from build123d import *

# Parameters (mm, degrees)
F0_W     = 40
F0_H     = 40
F1_DEPTH = 40.3
F2_W     = 25
F2_H     = 15
F3_DEPTH = 24.6
F6_W     = 20.776337
F6_H     = 21.012508
F7_DEPTH = 32
F8_R     = 7.245927
F8_R_2   = 6.636752
F8_R_3   = 8.331711
F8_R_4   = 4.708623
F9_DEPTH = 21.6


with BuildPart() as f1:
    # F0 (on Top) → F1 (new body)
    with BuildSketch(Plane.XY):
        with Locations((-31.879965, 27.884198)):
            Rectangle(F0_W, F0_H)
    extrude(amount=F1_DEPTH)

    # F2 (on face) → F3 (join)
    with BuildSketch(Plane.XZ.offset(-7.884198)):
        with Locations((-37.312957, 7.5)):
            Rectangle(F2_W, F2_H)
    extrude(amount=F3_DEPTH)

    # F6 (on face) → F7 (join)
    with BuildSketch(Plane.YZ.offset(-11.879965)):
        with Locations((27.700019, 16.992602)):
            Rectangle(F6_W, F6_H)
    extrude(amount=F7_DEPTH)

    # F8 (on face) → F9 (join)
    with BuildSketch(Plane.XY.offset(40.3)):
        with Locations((-43.442782, 35.17646)):
            Circle(F8_R)
        with Locations((-23.779849, 17.740337)):
            Circle(F8_R_2)
        with Locations((-25.526628, 37.980523)):
            Circle(F8_R_3)
        with Locations((-43.442782, 13.669529)):
            Circle(F8_R_4)
    extrude(amount=F9_DEPTH)


solid = f1.part
For this review, take the finished solid that the model builds, in its own axes (mm). A direction names the side the tool comes from. Give positions to 0.01 mm unless a question says otherwise; leave off trailing zeros. Loops run counter-clockwise (first coordinate to the right, second up) from the corner with the lowest first, then second, coordinate; pieces in that order, holes last. Notation, with made-up numbers: M -17.5,65.5 L 30.5,65.5 A24 cw 30.5,100.5 Z; hole C -36.5,-24.5 d6. An arc over 180 degrees is marked long. Put each result on its own line as item: value. Start each with the question number.
(1) Wall thickness on L1, parallel to Z at x = -33.5, y = 15.5; L2, parallel to X at y = 16, z = 21.5; L3, parallel to Y at x = -45.5, z = 24: over which ranges is each line inside the solid? List them lowest first.
(2) Add section C-C, the plane y = 16. Write out the cut boundary in (x, z), then the cut area to 3 significant figures.
(3) Add section B-B, the plane x = 8. Write out the cut boundary in (y, z), then the cut area to 3 significant figures.
(4) For pin 1 (23 mm diameter, centred on x = 10.5, y = 25, fed in from +Z); pin 2 (6 mm diameter, centred on y = 11, z = 49, fed in from -X); pin 3 (6.5 mm diameter, centred on x = 2, z = 21, fed in from -Y), all flat-tipped, find the tip position at first contact; note any pin that passes through.
(5) The part is to be moulded in two halves that separate along X. For faces 4 (the cylindrical face through (-36.53, 37.35, 50.95)), 5 (the flat face through (-32, 47.884, 20)), 6 (the flat face through (-49.813, -4, 7)), say which applies: +X half, -X half, draft (parallel to the pull), parting line (faces both ways), or undercut.
(6) Machinability: for faces 1 (the flat face through (4, 28, 27.499)), 2 (the flat face through (4, 28, 6.486)), 3 (the flat face through (-24.813, -4, 7)), which of the approach directions +Z, -Z, +X, -X, +Y, -Y give a long, thin tool a straight path to every point of the face, cutting with its end or side? Answer none if there is none.
(7) Add section A-A, the plane z = 18. Write out the cut boundary in (x, y), then the cut area to 3 significant figures.
(8) Add section D-D, the plane z = 54.5. Write out the cut boundary in (x, y).
Result:
1. L1: z = 0 to 40.3
1. L2: x = -51.88 to -11.88
1. L3: y = 7.88 to 47.88
2. outline: M -51.88,0 L -11.88,0 L -11.88,40.3 L -17.38,40.3 L -17.38,61.9 L -30.18,61.9 L -30.18,40.3 L -39.35,40.3 L -39.35,61.9 L -47.53,61.9 L -47.53,40.3 L -51.88,40.3 Z
2. area: 2,070 mm^2
3. outline: M 17.31,6.49 L 38.09,6.49 L 38.09,27.5 L 17.31,27.5 Z
3. area: 437 mm^2
4. pin 1: stops at z = 27.5
4. pin 2: stops at x = -48.15
4. pin 3: stops at y = 17.31
5. face 4: undercut
5. face 5: draft
5. face 6: -X half
6. face 1: +Z, +X, +Y, -Y
6. face 2: -Z, +X, +Y, -Y
6. face 3: +Z, -Z, +X, -Y
7. outline: M -51.88,7.88 L -11.88,7.88 L -11.88,17.31 L 20.12,17.31 L 20.12,38.09 L -11.88,38.09 L -11.88,47.88 L -51.88,47.88 Z
7. area: 2,260 mm^2
8. outline: C -43.44,35.18 d14.49; C -43.44,13.67 d9.42; C -25.53,37.98 d16.66; C -23.78,17.74 d13.27
